Build history of the part. All positions in model axes, mm. A direction names the side the tool comes from. Give positions to 0.01 mm unless a question says otherwise; leave off trailing zeros. One line per item, written item: value. Start each with the question number.
(1) Two-plate mould, pull along Z, no slides. Class faces 3 (the flat face through (5.5, 7, -64)), 4 (the flat face through (127, 0, -60)): +Z half, -Z half, draft (parallel to the pull), parting line (faces both ways), or undercut.
(2) Pin check, flat tips, straight feed: pin 1 (4 mm diameter, centred on y = 5.5, z = -59.5, fed in from +X); pin 2 (6.5 mm diameter, centred on y = 4, z = -70, fed in from -X); pin 3 (1.5 mm diameter, centred on y = 8.5, z = -20, fed in from +X). Stop position of each tip, or through.
(3) Which spindle directions (+Z, -Z, +X, -X, +Y, -Y) get a long thin tool onto all of the face, cutting with end or side? Do faces 1 (the flat face through (64, 7, -124.5)), 2 (the flat face through (1, 13, -59)). Say none if no direction does.
(4) Probe line 1 (Z direction, x = 42.5, y = 7); line 2 (X direction, y = 2.5, z = -122); line 3 (X direction, y = 10.5, z = -93). List the from-to ranges inside material, lowest first.
```python
from build123d import *

# Parameters (mm, degrees)
SKETCH1_W           = 130
SKETCH1_H           = 130
BOSS_EXTRUDE1_DEPTH = 13
BOSS_EXTRUDE1_TAPER = -45
SKETCH2_W           = 119
SKETCH2_H           = 119
CUT_EXTRUDE1_DEPTH  = 13


with BuildPart() as part:
    # Sketch1 → Boss-Extrude1 (new body)
    with BuildSketch(Plane(origin=(0, 0, 0), x_dir=(1, 0, 0), z_dir=(0, 1, 0))):
        with Locations((65, 65)):
            Rectangle(SKETCH1_W, SKETCH1_H)
    extrude(amount=BOSS_EXTRUDE1_DEPTH, taper=BOSS_EXTRUDE1_TAPER)

    # Sketch2 → Cut-Extrude1 (cut)
    with BuildSketch(Plane(origin=(0, 13, 0), x_dir=(1, 0, 0), z_dir=(0, 1, 0))):
        with Locations((65, 65)):
            Rectangle(SKETCH2_W, SKETCH2_H)
    extrude(amount=-CUT_EXTRUDE1_DEPTH, mode=Mode.SUBTRACT)


solid = part.part
```
Results below:
1. face 3: undercut
1. face 4: draft
2. pin 1: stops at x = 137.5
2. pin 2: stops at x = -7.25
2. pin 3: stops at x = 139.25
3. face 1: +Y, -Y
3. face 2: +Z, -Z, +X, -X, +Y
4. line 1: z = -137 to -124.5, -5.5 to 7
4. line 2: x = -2.5 to 5.5, 124.5 to 132.5
4. line 3: x = -10.5 to 5.5, 124.5 to 140.5
